Autodesk Inventor part; units mm, degrees
ref_plane "YZ Plane" through (0, 0, 0) normal (1, 0, 0) x (0, 1, 0)
ref_plane "XZ Plane" through (0, 0, 0) normal (0, 1, 0) x (-1, 0, 0)
ref_plane "XY Plane" through (0, 0, 0) normal (0, 0, 1) x (1, 0, 0)
sketch "Sketch1" plane through (0, 0, 0) normal (0, 0, 1) x (1, 0, 0)
  line L0 (0, 0) -> (49.5, 0)
  line L1 (49.5, 0) -> (49.5, 79)
  line L2 (49.5, 79) -> (0, 79)
  line L3 (0, 79) -> (0, 0)
  dimension "d0" = 49.5
  dimension "d1" = 79
extrude "Extrusion1" add sketch "Sketch1" along normal blind 2.5
sketch "Sketch2" plane through (0, 0, 0) normal (0, 0, 1) x (1, 0, 0)
  line L0 (0, 79) -> (0, 0)
  line L1 (49.5, 79) -> (0, 79)
  point P0 (12.777, 72.735)
  point P1 (36.551, 34.406)
  dimension "d4" = 12.777
  dimension "d5" = 6.265
  dimension "d6" = 38.329
  dimension "d7" = 23.774
hole "Hole1" at (12.777, 72.735, 0) at (36.551, 34.406, 0) direction (0, 0, 1) diameter 3.3 end through all
sketch "Sketch3" plane through (0, 0, 0) normal (0, 0, 1) x (1, 0, 0)
  line L0 (0, 0) -> (49.5, 0)
  line L1 (0, 79) -> (0, 0)
  point P0 (5.25, 6.25)
  point P1 (43.25, 6.25)
  point P2 (43.25, 72.75)
  point P3 (6.25, 72.75)
  dimension "d15" = 6.25
  dimension "d16" = 5.25
  dimension "d17" = 38
  dimension "d18" = 72.75
  dimension "d26" = 6.25
hole "Hole2" at (5.25, 6.25, 0) at (43.25, 6.25, 0) at (43.25, 72.75, 0) at (6.25, 72.75, 0) direction (0, 0, 1) diameter 3.3 end through all
properties part number "Tapadera_carcasa"
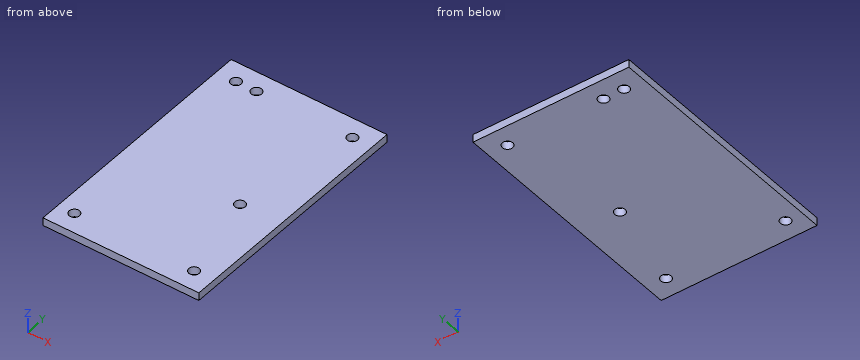
Build history of the part. All positions in model axes, mm. Round coordinates to 2 decimals unless told otherwise and drop trailing zeros. Write each loop counter-clockwise with the first axis right and the second up, starting at its lowest first coordinate (ties: lowest second). Pieces come first, ordered by that corner, then holes. Notation, with made-up numbers: (3.5, 74) -> (43.5, 74) arc R20 cw to (43.5, 84) -> close; hole circle Ø3 at (-24.75, 64.5). An arc over 180 degrees is marked (long way). Put each result on its own line as item: value.
Item 1: Flat gauge pin, fed straight in: P1, Ø5.5, axis at x = 36.551, y = 34.406, coming from the +Z side. Where does the tip first touch, or does it go through?
Here are the results:
P1: stops at z = 2.5
Item 2: Slice it at C-C, the plane y = 72.75. Give the cut face in (x, z), plus the area to 3 significant figures.
Here are the results:
outline: (0, 0) -> (4.6, 0) -> (4.6, 2.5) -> (0, 2.5) -> close; (7.9, 0) -> (11.13, 0) -> (11.13, 2.5) -> (7.9, 2.5) -> close; (14.43, 0) -> (41.6, 0) -> (41.6, 2.5) -> (14.43, 2.5) -> close; (44.9, 0) -> (49.5, 0) -> (49.5, 2.5) -> (44.9, 2.5) -> close
area: 99.0 mm^2
Item 3: Slice it at A-A, the plane y = 6.25. Give the cut face in (x, z).
Here are the results:
outline: (0, 0) -> (3.6, 0) -> (3.6, 2.5) -> (0, 2.5) -> close; (6.9, 0) -> (41.6, 0) -> (41.6, 2.5) -> (6.9, 2.5) -> close; (44.9, 0) -> (49.5, 0) -> (49.5, 2.5) -> (44.9, 2.5) -> close
Item 4: Slice it at B-B, the plane x = 43.25. Give the cut face in (y, z), plus the area to 3 significant figures.
Here are the results:
outline: (0, 0) -> (4.6, 0) -> (4.6, 2.5) -> (0, 2.5) -> close; (7.9, 0) -> (71.1, 0) -> (71.1, 2.5) -> (7.9, 2.5) -> close; (74.4, 0) -> (79, 0) -> (79, 2.5) -> (74.4, 2.5) -> close
area: 181 mm^2
Item 5: Wall check: probe 1 along Y at (x, z) = (43.25, 0.85); probe 2 along X at (y, z) = (72.75, 0.65); probe 3 along Y at (x, z) = (5.25, 0.9). Give the ranges that are in metal, low to high. Write a range as from..to.
Here are the results:
probe 1: y = 0..4.6, 7.9..71.1, 74.4..79
probe 2: x = 0..4.6, 7.9..11.13, 14.43..41.6, 44.9..49.5
probe 3: y = 0..4.6, 7.9..71.44, 74.06..79
